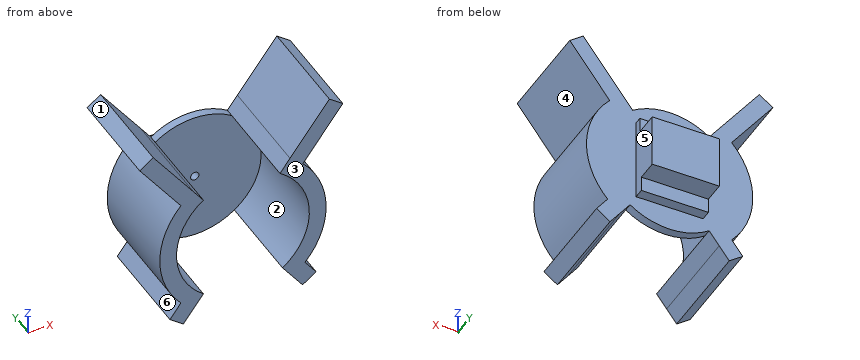
```python
from build123d import *

# Parameters (mm, degrees)
F1_DEPTH      = 38.1
F2_R          = 50.292
F3_DEPTH      = 38.1
F3_DEPTH_BACK = 31.75
F4_R          = 3.175
F5_DEPTH      = 38.101
F6_W          = 7.948064871
F6_H          = 11.407840997
F7_DEPTH      = 25.4


with BuildPart() as f1:
    # F0 (on Front) → F1 (new body, symmetric)
    with BuildSketch(Plane.XZ):
        with BuildLine():
            ThreePointArc((-39.1949844139, 31.5125127655), (-34.8668765946, 36.2434294809), (-29.972, 40.38520125))
            Line((-29.972, 40.38520125), (-37.5791103585, 50.55494564))
            ThreePointArc((-37.5791103585, 50.55494564), (-42.506880267, 46.4882479125), (-46.9973581988, 41.9432996596))
            Line((-46.9973581988, 41.9432996596), (-39.1949844139, 31.5125127655))
        make_face()
        with BuildLine():
            ThreePointArc((-46.9973581988, 41.9432996596), (-42.506880267, 46.4882479125), (-37.5791103585, 50.55494564))
            Line((-37.5791103585, 50.55494564), (-68.0073361401, 91.2336349005))
            Line((-68.0073361401, 91.2336349005), (-78.1770228702, 83.6265676724))
            Line((-78.1770228702, 83.6265676724), (-46.9973581988, 41.9432996596))
        make_face()
        with BuildLine():
            ThreePointArc((35.649530109, 51.9336409951), (40.7121086164, 48.067829949), (45.3583906555, 43.7105074455))
            Line((45.3583906555, 43.7105074455), (75.6600814431, 84.2200354233))
            Line((75.6600814431, 84.2200354233), (65.490394713, 91.8271026513))
            Line((65.490394713, 91.8271026513), (35.649530109, 51.9336409951))
        make_face()
        with BuildLine():
            Line((46.9973581988, -41.9432996596), (39.1949844139, -31.5125127655))
            ThreePointArc((39.1949844139, -31.5125127655), (34.8668765946, -36.2434294809), (29.972, -40.38520125))
            Line((29.972, -40.38520125), (37.5791103585, -50.55494564))
            ThreePointArc((37.5791103585, -50.55494564), (42.506880267, -46.4882479125), (46.9973581988, -41.9432996596))
        make_face()
        with BuildLine():
            Line((55.3558211861, -53.1175074821), (46.9973581988, -41.9432996596))
            ThreePointArc((46.9973581988, -41.9432996596), (42.506880267, -46.4882479125), (37.5791103585, -50.55494564))
            Line((37.5791103585, -50.55494564), (45.186134456, -60.7245747102))
            Line((45.186134456, -60.7245747102), (55.3558211861, -53.1175074821))
        make_face()
        with BuildLine():
            Line((-37.5791103585, -50.55494564), (-29.972, -40.38520125))
            ThreePointArc((-29.972, -40.38520125), (-34.8668765946, -36.2434294809), (-39.1949844139, -31.5125127655))
            Line((-39.1949844139, -31.5125127655), (-46.9973581988, -41.9432996596))
            ThreePointArc((-46.9973581988, -41.9432996596), (-42.506880267, -46.4882479125), (-37.5791103585, -50.55494564))
        make_face()
        with BuildLine():
            Line((-45.186134456, -60.7245747102), (-37.5791103585, -50.55494564))
            ThreePointArc((-37.5791103585, -50.55494564), (-42.506880267, -46.4882479125), (-46.9973581988, -41.9432996596))
            Line((-46.9973581988, -41.9432996596), (-55.3558211861, -53.1175074821))
            Line((-55.3558211861, -53.1175074821), (-45.186134456, -60.7245747102))
        make_face()
        with BuildLine():
            ThreePointArc((28.0345791239, 41.7534146789), (33.0960785887, 37.867332175), (37.624745303, 33.3716017728))
            Line((37.624745303, 33.3716017728), (45.3583906555, 43.7105074455))
            ThreePointArc((45.3583906555, 43.7105074455), (40.7121086164, 48.067829949), (35.649530109, 51.9336409951))
            Line((35.649530109, 51.9336409951), (28.0345791239, 41.7534146789))
        make_face()
        with BuildLine():
            ThreePointArc((-39.1949844139, -31.5125127655), (-50.292, 0), (-39.1949844139, 31.5125127655))
            Line((-39.1949844139, 31.5125127655), (-46.9973581988, 41.9432996596))
            ThreePointArc((-46.9973581988, 41.9432996596), (-62.992, 0), (-46.9973581988, -41.9432996596))
            Line((-46.9973581988, -41.9432996596), (-39.1949844139, -31.5125127655))
        make_face()
        with BuildLine():
            ThreePointArc((37.624745303, 33.3716017728), (47.0186609485, 17.8474308126), (50.292, 0))
            ThreePointArc((50.292, 0), (47.4366916012, -16.704656654), (39.1949844139, -31.5125127655))
            Line((39.1949844139, -31.5125127655), (46.9973581988, -41.9432996596))
            ThreePointArc((46.9973581988, -41.9432996596), (58.8576658204, -22.444759704), (62.992, 0))
            ThreePointArc((62.992, 0), (58.4174965578, 23.5666747742), (45.3583906555, 43.7105074455))
            Line((45.3583906555, 43.7105074455), (37.624745303, 33.3716017728))
        make_face()
        with BuildLine():
            ThreePointArc((39.1949844139, -31.5125127655), (47.4366916012, -16.704656654), (50.292, 0))
            ThreePointArc((50.292, 0), (47.0186609485, 17.8474308126), (37.624745303, 33.3716017728))
            ThreePointArc((37.624745303, 33.3716017728), (33.0960785887, 37.867332175), (28.0345791239, 41.7534146789))
            ThreePointArc((28.0345791239, 41.7534146789), (-1.1859181715, 50.2780156936), (-29.972, 40.38520125))
            ThreePointArc((-29.972, 40.38520125), (-34.8668765946, 36.2434294809), (-39.1949844139, 31.5125127655))
            ThreePointArc((-39.1949844139, 31.5125127655), (-50.292, 0), (-39.1949844139, -31.5125127655))
            ThreePointArc((-39.1949844139, -31.5125127655), (-34.8668765946, -36.2434294809), (-29.972, -40.38520125))
            ThreePointArc((-29.972, -40.38520125), (0, -50.292), (29.972, -40.38520125))
            ThreePointArc((29.972, -40.38520125), (34.8668765946, -36.2434294809), (39.1949844139, -31.5125127655))
        make_face()
    extrude(amount=F1_DEPTH, both=True)

    # F2 (on Front) → F3 (cut, two sides)
    with BuildSketch(Plane.XZ) as f3_sk:
        Circle(F2_R)
    extrude(amount=F3_DEPTH, mode=Mode.SUBTRACT)
    extrude(f3_sk.sketch, amount=-F3_DEPTH_BACK, mode=Mode.SUBTRACT)

    # F4 (on Front) → F5 (cut, through all)
    with BuildSketch(Plane.XZ):
        Circle(F4_R)
    extrude(amount=-F5_DEPTH, mode=Mode.SUBTRACT)

    # F6 (on Right) → F7 (join, symmetric)
    with BuildSketch(Plane.YZ):
        Polygon((37.9081480205, 31.9281220436), (37.8097093926, 20.3845500946), (43.4490628541, 20.3845500946), (43.547091421, 31.8800355541), align=None)
        Polygon((43.4490628541, 20.3845500946), (37.8097093926, 20.3845500946), (37.8097093926, -20.3845500946), (45.7577742636, -20.3845500946), (61.4949830113, -20.3845500946), (61.4949830113, 20.3845500946), align=None)
        with Locations((41.7837418281, -26.0884705931)):
            Rectangle(F6_W, F6_H)
    extrude(amount=F7_DEPTH, both=True)


solid = f1.part
```
Input: part model. Units: mm. Frame: model coordinates. Face numbers are marked on the shaded views. A direction names the side the tool comes from. Round coordinates to 2 decimals unless told otherwise and drop trailing zeros. Loops run counter-clockwise (first coordinate to the right, second up) from the corner with the lowest first, then second, coordinate; pieces in that order, holes last. Notation, with made-up numbers: (-9, -30) -> (-4, -30) arc R11 cw to (-4, -10) -> close; hole circle Ø8 at (72, 16). An arc over 180 degrees is marked (long way). Use one line per item in the form item = value. Start each with the question number.
Item 1: Material intervals for L1, parallel to Z at x = 0, y = 34.5 (3 decimals); L2, parallel to Y at x = 68.5, z = 78.5; L3, parallel to Y at x = -29, z = -14.5, sorted ascending. Write a range as from..to.
Item 2: Set-up query: the marked faces 4, 5 and 6. Return all of +Z, -Z, +X, -X, +Y, -Y with unobstructed straight access to the full face (end or side cutting, diameter ignored); none if empty.
Item 3: Section query B-B on z = 0. Return the cut outline in (x, y) (3 decimals).
Item 4: Contact query for flat-ended pins moving along their axis: pin 1 Ø6 at (x, z) = (13.5, -36.5) entering from +Y; pin 2 Ø6 at (x, y) = (51, 38) entering from -Z; pin 3 Ø18.5 at (y, z) = (52.5, 7) entering from +X. Output: stop coordinate, or through.
Item 5: Section query A-A on y = 13. Return the cut outline in (x, z), then the cut area to 3 significant figures.
Item 6: Section query C-C on x = 0. Return the cut outline in (y, z) (3 decimals).
Item 7: Mould query, pull axis Z, two halves, no side actions, for the marked faces 1, 2 and 3. Classes: pulls with the +Z half, pulls with the -Z half, needs draft (parallel to the pull), parting line crosses it, or undercut.
Item 8: Section query D-D on z = 58. Return the cut outline in (x, y).
Ans:
q1.L1 = -50.292..-3.175, 3.175..50.292
q1.L2 = -38.1..38.1
q1.L3 = 31.75..38.1
q2.face_4 = +X, +Y, -Y
q2.face_5 = +Z, -Z, +X, +Y
q2.face_6 = -X, +Y, -Y
q3.outline = (-62.992, -38.1) -> (-50.292, -38.1) -> (-50.292, 31.75) -> (-3.175, 31.75) -> (-3.175, 37.81) -> (3.175, 37.81) -> (3.175, 31.75) -> (50.292, 31.75) -> (50.292, -38.1) -> (62.992, -38.1) -> (62.992, 38.1) -> (25.4, 38.1) -> (25.4, 61.495) -> (-25.4, 61.495) -> (-25.4, 38.1) -> (-62.992, 38.1) -> close
q4.pin_1 = 38.1
q4.pin_2 = -58.62
q4.pin_3 = 25.4
q5.outline = (-78.18, 83.63) -> (-47, 41.94) arc R62.99 ccw to (-47, -41.94) -> (-55.36, -53.12) -> (-45.19, -60.72) -> (-29.97, -40.39) arc R50.29 cw to (-29.97, 40.39) -> (-68.01, 91.23) -> close; (28.03, 41.75) arc R50.29 cw to (29.97, -40.39) -> (45.19, -60.72) -> (55.36, -53.12) -> (47, -41.94) arc R62.99 ccw to (45.36, 43.71) -> (75.66, 84.22) -> (65.49, 91.83) -> close
q5.area = 4,330 mm^2
q6.outline = (31.75, -50.292) -> (38.1, -50.292) -> (38.1, -31.792) -> (45.758, -31.792) -> (45.758, -20.385) -> (61.495, -20.385) -> (61.495, 20.385) -> (43.449, 20.385) -> (43.547, 31.88) -> (38.1, 31.926) -> (38.1, 50.292) -> (31.75, 50.292) -> (31.75, 3.175) -> (37.81, 3.175) -> (37.81, -3.175) -> (31.75, -3.175) -> close
q7.face_1 = pulls with the +Z half
q7.face_2 = undercut
q7.face_3 = needs draft
q8.outline = (-59.01, -38.1) -> (-43.15, -38.1) -> (-43.15, 38.1) -> (-59.01, 38.1) -> close; (40.19, -38.1) -> (56.05, -38.1) -> (56.05, 38.1) -> (40.19, 38.1) -> close
